from build123d import *

# Parameters (mm, degrees)
F1_DEPTH = 38.1
F2_R     = 3.175
F4_DEPTH = 38.1


with BuildPart() as f1:
    # F0 (on Front) → F1 (new body)
    with BuildSketch(Plane.XZ):
        Polygon((13.198227, 22.86), (-13.198227, 22.86), (-26.396454, 0), (-13.198227, -22.86), (13.198227, -22.86), (26.396454, 0), align=None)
    extrude(amount=F1_DEPTH)

    # F2
    f2_edges = [f1.edges().sort_by_distance(p)[0] for p in [
        (13.198227, -19.05, 22.86),
        (26.396454, -19.05, 0),
        (13.198227, -19.05, -22.86),
        (-13.198227, -19.05, -22.86),
        (-26.396454, -19.05, 0),
        (-13.198227, -19.05, 22.86),
    ]]
    fillet(f2_edges, radius=F2_R)

    # F3 (on face) → F4 (cut, through all)
    with BuildSketch(Plane.XZ.offset(38.1)):
        with BuildLine():
            ThreePointArc((0, 8.89), (-4.490128, -1.950128), (6.35, 2.54))
            ThreePointArc((6.35, 2.54), (4.490128, 7.030128), (0, 8.89))
        make_face()
    extrude(amount=-F4_DEPTH, mode=Mode.SUBTRACT)


solid = f1.part
Could you check a few things on this model? Use its own coordinates, in mm. Coordinates: 2 decimals unless noted, no trailing zeros. Loops run counter-clockwise (first coordinate to the right, second up) from the corner with the lowest first, then second, coordinate; pieces in that order, holes last.
1. For P1, Ø16.5, axis at x = 0, z = 2.54, coming from the -Y side; P2, Ø2, axis at x = 14.5, y = -15.5, coming from the -Z side; P3, Ø1, axis at y = -29, z = 8.5, coming from the +X side; P4, Ø4, axis at y = -6, z = -10.5, coming from the -X side, each with a flat end and sliding along its axis, tell me the tip position at first contact or that it passes through.
2. We'd pull the mould along Y, two halves only. Please class faces 1 (the face through (0, -38.1, -5)), 2 (the face through (0, 0, -5)), 3 (the face through (-19.7, -18.8, 11.6)): released by +Y, released by -Y, zero draft, split by the parting line, or undercut.
3. Imagine slicing it at D-D (z = -9). Please give me the cut outline in (x, y), and give its area (3 significant figures).
4. Imagine slicing it at C-C (x = 4). Please give me the cut outline in (y, z), and give its area (3 significant figures).
5. I need wall thicknesses on L1, parallel to X at y = -18, z = 2.54; L2, parallel to X at y = -32, z = 7 (3 decimals); L3, parallel to X at y = -11, z = -20.5. Which ranges of each line are inside material? Lowest first, please.
6. Imagine slicing it at B-B (z = 4). Please give me the cut outline in (x, y), and give its area (3 significant figures).
Computed values:
1. P1: stops at y = -38.1
1. P2: stops at z = -22.04
1. P3: stops at x = 21.78
1. P4: stops at x = -21.49
2. face 1: released by -Y
2. face 2: released by +Y
2. face 3: zero draft
3. outline: (-21.2, -38.1) - (21.2, -38.1) - (21.2, 0) - (-21.2, 0) - close
3. area: 1,620 mm2
4. outline: (-38.1, -22.86) - (0, -22.86) - (0, -2.39) - (-38.1, -2.39) - close; (-38.1, 7.47) - (0, 7.47) - (0, 22.86) - (-38.1, 22.86) - close
4. area: 1,370 mm2
5. L1: x = -24.93 to -6.35, 6.35 to 24.93
5. L2: x = -22.355 to -4.52, 4.52 to 22.355
5. L3: x = -14.56 to 14.56
6. outline: (-24.09, -38.1) - (-6.18, -38.1) - (-6.18, 0) - (-24.09, 0) - close; (6.18, -38.1) - (24.09, -38.1) - (24.09, 0) - (6.18, 0) - close
6. area: 1,360 mm2
